The model under review builds one solid part; all positions refer to its coordinate system, in mm. A direction names the side the tool comes from. Round coordinates to 2 decimals unless told otherwise and drop trailing zeros. Loops run counter-clockwise (first coordinate to the right, second up) from the corner with the lowest first, then second, coordinate; pieces in that order, holes last. Notation, with made-up numbers: (84, 34) -> (137, 34) arc R18 cw to (137, 51) -> close; hole circle Ø3 at (-3, 27). An arc over 180 degrees is marked (long way). Use a Markdown table: item, result. Add a question column.
1) Consider section C-C on x = 27.5. Give the boundary of the cut face in (y, z).
2) Insertion check: pin 1 (0.9 mm diameter, centred on y = 28, z = 1.5, fed in from -X); pin 2 (0.9 mm diameter, centred on x = 26, z = 2, fed in from +Y); pin 3 (0.9 mm diameter, centred on x = 50, z = 1, fed in from -Y). Each pin has a flat end and moves straight along its axis. Give the tip position at first contact, or say it passes through.
3) Wall thickness on probe 1 along X at (y, z) = (5, 0.95); probe 2 along X at (y, z) = (11, 1.1); probe 3 along Y at (x, z) = (0.5, 0.2): over which ranges is each line inside the solid? List them lowest first.
4) Consider section D-D on y = 29. Give the boundary of the cut face in (x, z), plus the area to 3 significant figures.
5) For faces 5 (the flat face through (51, 30, 1)), 6 (the flat face through (3, 30, 1)), 7 (the flat face through (33, 32, 1)), 8 (the flat face through (48.8, -2, 1)), list the 3-axis set-ups (+Z, -Z, +X, -X, +Y, -Y) from which the entire face can be reached by the end or side of a thin tool; tool diameter is ignored.
6) Consider section A-A on y = 2. Give the boundary of the cut face in (x, z).
7) Mouldability with a two-part tool opening along Y and no side actions: class faces 1 (the flat face through (-3.1, 15, 1)), 2 (the flat face through (27, 30, 1)), 3 (the cylindrical face through (10.8, 8.6, 1.5)), 4 (the flat face through (-2, 7.1, 1)) as released by +Y, released by -Y, zero draft, split by the parting line, or undercut.
from build123d import *

# Parameters (mm, degrees)
SKETCH1_R           = 2.525
BOSS_EXTRUDE1_DEPTH = 3


with BuildPart() as part:
    # Sketch1 → Boss-Extrude1 (new body)
    with BuildSketch(Plane.XY):
        Polygon((5, 30), (0, 30), (0, 22.9), (-3.1, 22.9), (-3.1, 7.1), (0, 7.1), (0, 0), (5, 0), (5, -3), (15.9, -3), (15.9, 7), (37.9, 7), (37.9, -3), (48.8, -3), (48.8, 0), (53.8, 0), (53.8, 7.1), (56.9, 7.1), (56.9, 22.9), (53.8, 22.9), (53.8, 30), (48.8, 30), (48.8, 33), (33, 33), (33, 30), (20.8, 30), (20.8, 33), (5, 33), align=None)
        with Locations((9.620987069, 10.833243053)):
            Circle(SKETCH1_R, mode=Mode.SUBTRACT)
    extrude(amount=BOSS_EXTRUDE1_DEPTH)


solid = part.part
Result set:
| question | item | result |
|---|---|---|
| 1 | outline | (7, 0) -> (30, 0) -> (30, 3) -> (7, 3) -> close |
| 2 | pin 1 | x = 0 |
| 2 | pin 2 | y = 30 |
| 2 | pin 3 | y = 0 |
| 3 | probe 1 | 0 to 15.9, 37.9 to 53.8 |
| 3 | probe 2 | -3.1 to 7.1, 12.14 to 56.9 |
| 3 | probe 3 | 0 to 30 |
| 4 | outline | (0, 0) -> (53.8, 0) -> (53.8, 3) -> (0, 3) -> close |
| 4 | area | 161 mm2 |
| 5 | face 5 | +Z, -Z, +X, +Y |
| 5 | face 6 | +Z, -Z, -X, +Y |
| 5 | face 7 | +Z, -Z, +Y |
| 5 | face 8 | +Z, -Z, +X, -Y |
| 6 | outline | (0, 0) -> (15.9, 0) -> (15.9, 3) -> (0, 3) -> close; (37.9, 0) -> (53.8, 0) -> (53.8, 3) -> (37.9, 3) -> close |
| 7 | face 1 | zero draft |
| 7 | face 2 | released by +Y |
| 7 | face 3 | undercut |
| 7 | face 4 | released by -Y |
